Geometry check sheet. Reference: the model listing, model coordinates, mm. Face numbers are marked on the shaded views. A direction names the side the tool comes from. Round coordinates to 2 decimals unless told otherwise and drop trailing zeros. Order: outer loops, then holes, each group sorted by start corner. A loop starts at its lowest first (then second) coordinate and runs counter-clockwise, first axis right, second up. Notation, with made-up numbers: (82.5, -24) - (107.5, -24) arc R12 cw to (107.5, -9) - close; hole circle Ø1 at (63, 25.5). An arc over 180 degrees is marked (long way). Write each question's results on one line, items separated by ' | '.
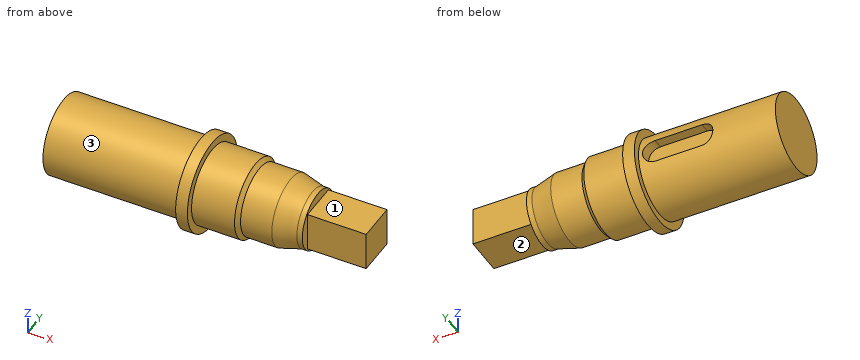
```python
from build123d import *

# Parameters (mm, degrees)
SKETCH_2_OUTSIDE_W   = 43.38
SKETCH_2_OUTSIDE_H   = 43.38
SKETCH_2_OUTSIDE_W_2 = 10
SKETCH_2_OUTSIDE_H_2 = 10
CUT_EXTRUDE_1_DEPTH  = 15
CUT_EXTRUDE_START    = 7
CUT_EXTRUDE_2_DEPTH  = 6


with BuildPart() as part:
    # Эскиз1 → Повернуть1 (revolve)
    with BuildSketch(Plane.XY):
        Polygon((-25, 10), (10, 10), (10, 12), (13, 12), (13, 10), (24, 10), (25, 9), (33, 9), (38.598076211, 7.5), (55, 7.5), (55, 0), (-25, 0), align=None)
    revolve(axis=Axis((0, 0, 0), (-1, 0, 0)))

    # Эскиз2 outside → Вырез-Вытянуть1 (cut)
    with BuildSketch(Plane(origin=(55, 0, 0), x_dir=(0, 0, -1), z_dir=(1, 0, 0))):
        Rectangle(SKETCH_2_OUTSIDE_W, SKETCH_2_OUTSIDE_H)
        Rectangle(SKETCH_2_OUTSIDE_W_2, SKETCH_2_OUTSIDE_H_2, mode=Mode.SUBTRACT)
    extrude(amount=-CUT_EXTRUDE_1_DEPTH, mode=Mode.SUBTRACT)

    # Эскиз3 → Вырез-Вытянуть2 (cut, through all)
    with BuildSketch(Plane(origin=(0, 0, 0), x_dir=(1, 0, 0), z_dir=(0, 1, 0)).offset(CUT_EXTRUDE_START)):
        with BuildLine():
            Line((-6, 3), (6, 3))
            ThreePointArc((6, 3), (9, 0), (6, -3))
            Line((6, -3), (-6, -3))
            ThreePointArc((-6, -3), (-9, 0), (-6, 3))
        make_face()
    extrude(amount=CUT_EXTRUDE_2_DEPTH, mode=Mode.SUBTRACT)


solid = part.part
```
(1) Depth check by flat-ended pin: pin 1 Ø3 at (x, z) = (-4, 0.5) entering from +Y; pin 2 Ø1.5 at (y, z) = (2, -7) entering from +X; pin 3 Ø2 at (x, z) = (25.5, 9) entering from -Y. Enter the tip coordinate at first touch or a pass-through.
Answers follow:
pin 1: y = 7 | pin 2: x = 40 | pin 3: y = -4.12
(2) Material ranges on line 1 (Y direction, x = 25, z = -5); line 2 (Y direction, x = 44, z = -1); line 3 (Z direction, x = -14, y = -0.25), recorded low to high.
Answers follow:
line 1: -7.48 to 7.48 | line 2: -5 to 5 | line 3: -10 to 10
(3) Section check B-B (x = -10.5). Record the cut outline in (y, z).
Answers follow:
outline: circle Ø20 at (0, 0)
(4) Access from +Z, -Z, +X, -X, +Y, -Y to the whole of each face (thin tool, end or side, straight path). Record for the marked faces 1, 2 and 3.
Answers follow:
face 1: +Z, +X, +Y, -Y | face 2: -Z, +X, +Y, -Y | face 3: -X
(5) Section check A-A (z = 0). Record the cut outline in (x, y).
Answers follow:
outline: (-25, -10) - (10, -10) - (10, -12) - (13, -12) - (13, -10) - (24, -10) - (25, -9) - (33, -9) - (38.6, -7.5) - (40, -7.5) - (40, -5) - (55, -5) - (55, 5) - (40, 5) - (40, 7.5) - (38.6, 7.5) - (33, 9) - (25, 9) - (24, 10) - (13, 10) - (13, 12) - (10, 12) - (10, 10) - (9, 10) - (9, 7) - (-9, 7) - (-9, 10) - (-25, 10) - close
(6) Section check C-C (x = 44). Record the cut outline in (y, z), then the cut area to 3 significant figures.
Answers follow:
outline: (-5, -5) - (5, -5) - (5, 5) - (-5, 5) - close | area: 100 mm²
